Check sheet for the modelled part. Datum: model origin and axes. Units: mm. A direction names the side the tool comes from. Round coordinates to 2 decimals unless told otherwise and drop trailing zeros. Write each loop counter-clockwise with the first axis right and the second up, starting at its lowest first coordinate (ties: lowest second). Pieces come first, ordered by that corner, then holes.
Item 1: Section check C-C, the plane x = -2. Record the cut outline in (y, z).
Item 2: Release check for a two-part mould opening along Y. For faces 1 (the flat face through (-15.865, -17.046, 0.74)), 2 (the cylindrical face through (-3.06, -16.4, 0.74)), 3 (the cylindrical face through (-29.752, 11.923, 0.74)), 4 (the cylindrical face through (3.11, -0.13, 0.74)) record: pulls with the +Y half, pulls with the -Y half, needs draft (parallel to the pull), parting line crosses it, or undercut.
Item 3: Material ranges on line 1 along Y through (x, z) = (-2.5, 1.3); line 2 along Y through (x, z) = (-1, 1.4); line 3 along X through (y, z) = (0, 0.65), recorded low to high.
Item 4: Section check B-B, the plane y = 0. Record the cut outline in (x, z).
Item 5: Section check D-D, the plane x = -25.75. Record the cut outline in (y, z), plus the area to 3 significant figures.
Item 6: Set-up check for faces 5 (the flat face through (-15.553, 17.141, 0.74)), 6 (the flat face through (-26, 4, 1)): record each of +Z, -Z, +X, -X, +Y, -Y from which the full face is reachable in a straight line by a thin tool's end or side.
Item 7: Section check A-A, the plane z = 0.9. Record the cut outline in (x, y) (3 decimals), plus the area to 3 significant figures.
from build123d import *

# Parameters (mm, degrees)
BOSS_EXTRUDE1_DEPTH   = 1.5
IZIM1_R               = 4.125
KES_EKSTR_ZYON1_DEPTH = 5


with BuildPart() as part:
    # Sketch1 → Boss-Extrude1 (new body)
    with BuildSketch(Plane.XY):
        with BuildLine():
            Line((-4.586520611, 20.5), (-26.831876879, 13.6870336))
            ThreePointArc((-26.831876879, 13.6870336), (-29.786221501, 11.888574472), (-31.518862928, 8.895154845))
            ThreePointArc((-31.518862928, 8.895154845), (-32.75, 0), (-31.518862928, -8.895154845))
            ThreePointArc((-31.518862928, -8.895154845), (-29.786221501, -11.888574472), (-26.831876879, -13.6870336))
            Line((-26.831876879, -13.6870336), (-4.586520611, -20.5))
            ThreePointArc((-4.586520611, -20.5), (4.125457599, -17.942905427), (5.211648434, -8.928611974))
            ThreePointArc((5.211648434, -8.928611974), (3.108013658, 0), (5.211648434, 8.928611974))
            ThreePointArc((5.211648434, 8.928611974), (4.125457599, 17.942905427), (-4.586520611, 20.5))
        make_face()
        with BuildLine():
            Line((-23.688447187, 4), (-27.811552813, 4))
            ThreePointArc((-27.811552813, 4), (-25.75, -4.5), (-23.688447187, 4))
        make_face(mode=Mode.SUBTRACT)
    extrude(amount=BOSS_EXTRUDE1_DEPTH)

    # Çizim1 → Kes-Ekstrüzyon1 (cut, symmetric)
    with BuildSketch(Plane(origin=(0, 0, 0), x_dir=(-1, 0, 0), z_dir=(0, 0, -1))):
        with Locations(Location((2.524172848, -12.31, 0), (0, 0, 180))):
            Circle(IZIM1_R)
        with Locations(Location((2.524172848, 12.31, 0), (0, 0, 180))):
            Circle(IZIM1_R)
    extrude(amount=KES_EKSTR_ZYON1_DEPTH, both=True, mode=Mode.SUBTRACT)


solid = part.part
Values found:
1. outline: (-20.86, 0) - (-16.4, 0) - (-16.4, 1.5) - (-20.86, 1.5) - close; (-8.22, 0) - (8.22, 0) - (8.22, 1.5) - (-8.22, 1.5) - close; (16.4, 0) - (20.86, 0) - (20.86, 1.5) - (16.4, 1.5) - close
2. face 1: pulls with the -Y half
2. face 2: undercut
2. face 3: pulls with the +Y half
2. face 4: undercut
3. line 1: y = -20.86 to -16.43, -8.19 to 8.19, 16.43 to 20.86
3. line 2: y = -20.78 to -16.14, -8.48 to 8.48, 16.14 to 20.78
3. line 3: x = -32.75 to -30.25, -21.25 to 3.11
4. outline: (-32.75, 0) - (-30.25, 0) - (-30.25, 1.5) - (-32.75, 1.5) - close; (-21.25, 0) - (3.11, 0) - (3.11, 1.5) - (-21.25, 1.5) - close
5. outline: (-14.02, 0) - (-4.5, 0) - (-4.5, 1.5) - (-14.02, 1.5) - close; (4, 0) - (14.02, 0) - (14.02, 1.5) - (4, 1.5) - close
5. area: 29.3 mm2
6. face 5: +Z, -Z, -X, +Y
6. face 6: +Z, -Z
7. outline: (-31.519, -8.895) arc R7 ccw to (-26.832, -13.687) - (-4.587, -20.5) arc R8.25 ccw to (5.212, -8.929) arc R20 cw to (5.212, 8.929) arc R8.25 ccw to (-4.587, 20.5) - (-26.832, 13.687) arc R7 ccw to (-31.519, 8.895) arc R32.75 ccw to start; hole (-27.812, 4) arc R4.5 ccw (long way) to (-23.688, 4) - close; hole circle Ø8.25 at (-2.524, -12.31); hole circle Ø8.25 at (-2.524, 12.31)
7. area: 1,090 mm2
